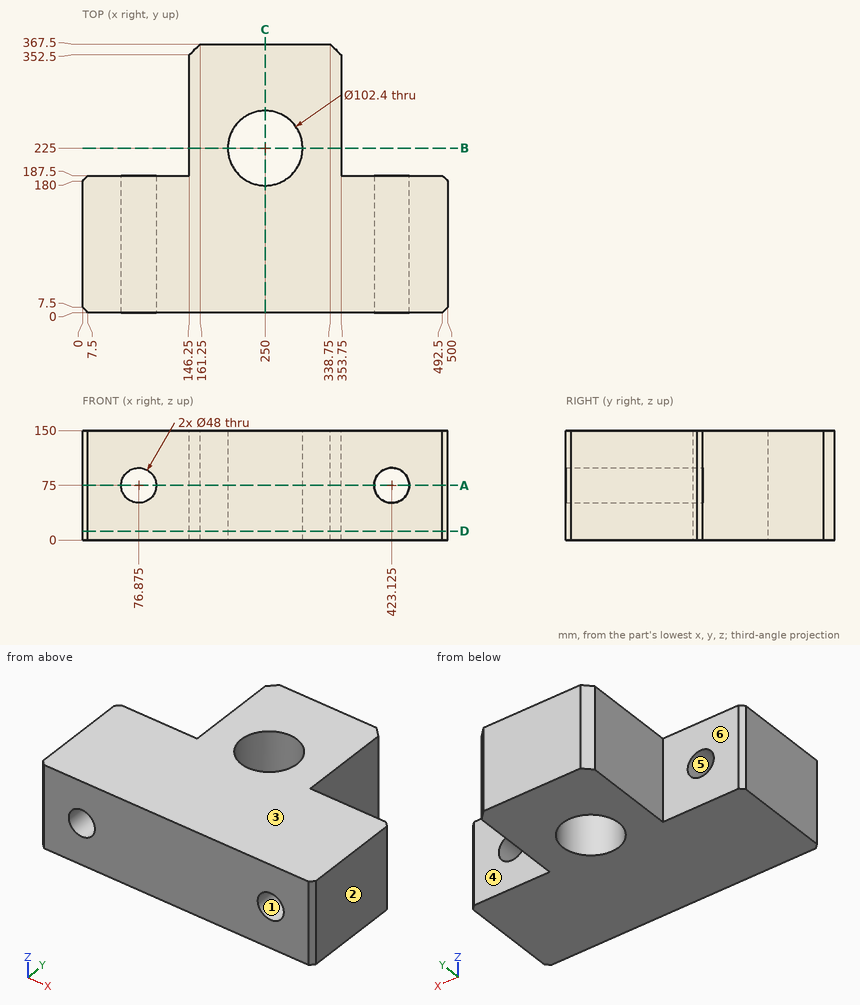
Part print with two shaded views. Sizes in mm from the minimum x, y, z corner. A direction names the side the tool comes from. Give positions to 0.01 mm unless a question says otherwise; leave off trailing zeros. Order: outer loops, then holes, each group sorted by start corner. A loop starts at its lowest first (then second) coordinate and runs counter-clockwise, first axis right, second up. Notation, with made-up numbers: M -6.5,18 L 14.5,18 A14 ccw 14.5,36 Z; hole C 19.25,68 d7. An arc over 180 degrees is marked long. Put each result on its own line as item: value.
Item 1: Cut at C-C on x = 250. Write the cut outline in (y, z).
Results are:
outline: M 0,0 L 173.8,0 L 173.8,150 L 0,150 Z; M 276.2,0 L 367.5,0 L 367.5,150 L 276.2,150 Z
Item 2: Cut at A-A on z = 75. Write the cut outline in (x, y) (3 decimals).
Results are:
outline: M 0,7.5 L 7.5,0 L 52.875,0 L 52.875,187.5 L 7.5,187.5 L 0,180 Z; M 100.875,0 L 399.125,0 L 399.125,187.5 L 353.75,187.5 L 353.75,352.5 L 338.75,367.5 L 161.25,367.5 L 146.25,352.5 L 146.25,187.5 L 100.875,187.5 Z; M 447.125,0 L 492.5,0 L 500,7.5 L 500,180 L 492.5,187.5 L 447.125,187.5 Z; hole C 250,225 d102.4
Item 3: Which spindle directions (+Z, -Z, +X, -X, +Y, -Y) get a long thin tool onto all of the face, cutting with end or side? Do the marked faces 4, 5 and 6. Say none if no direction does.
Results are:
face 4: +Z, -Z, +X, +Y
face 5: +Y, -Y
face 6: +Z, -Z, -X, +Y
Item 4: Wall check: probe 1 along X at (y, z) = (117, 75) (3 decimals); probe 2 along Y at (x, z) = (250, 100); probe 3 along X at (y, z) = (42.5, 83.5). Give the ranges that are in metal, low to high.
Results are:
probe 1: 0 to 52.875, 100.875 to 399.125, 447.125 to 500
probe 2: 0 to 173.8, 276.2 to 367.5
probe 3: 0 to 54.43, 99.32 to 400.68, 445.57 to 500
Item 5: Drop a flat-ended pin along its axis: pin 1 Ø1.5 at (y, z) = (240.5, 128) entering from -X. Give the stop position or say it passes through.
Results are:
pin 1: x = 146.25
Item 6: Pull direction Z, two halves, no side cores. Call the marked faces 1, 2 and 3: +Z half, -Z half, draft (parallel to the pull), parting line (faces both ways), or undercut.
Results are:
face 1: undercut
face 2: draft
face 3: +Z half
Item 7: Cut at D-D on z = 12.5. Write the cut outline in (x, y), then the cut area to 3 significant figures.
Results are:
outline: M 0,7.5 L 7.5,0 L 492.5,0 L 500,7.5 L 500,180 L 492.5,187.5 L 353.75,187.5 L 353.75,352.5 L 338.75,367.5 L 161.25,367.5 L 146.25,352.5 L 146.25,187.5 L 7.5,187.5 L 0,180 Z; hole C 250,225 d102.4
area: 123,000 mm2
Item 8: Cut at B-B on y = 225. Write the cut outline in (x, z).
Results are:
outline: M 146.25,0 L 198.8,0 L 198.8,150 L 146.25,150 Z; M 301.2,0 L 353.75,0 L 353.75,150 L 301.2,150 Z
